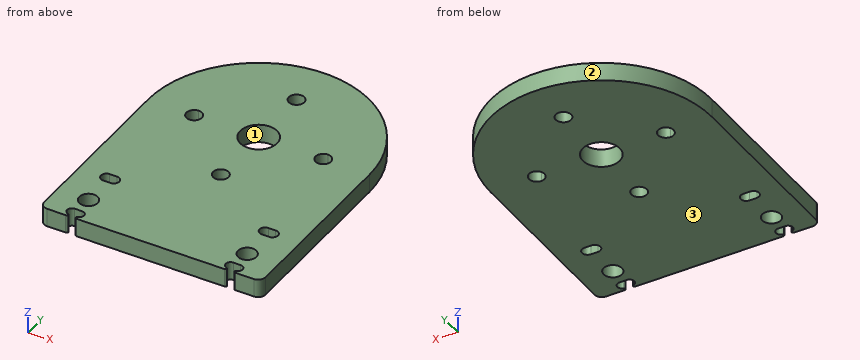
```python
from build123d import *

# Parameters (mm, degrees)
SKETCH1_R           = 2.5
BOSS_EXTRUDE1_DEPTH = 2.5
SKETCH2_R           = 5
CUT_EXTRUDE1_DEPTH  = 5
FILLET1_R           = 0.5
FILLET2_R           = 2


with BuildPart() as part:
    # Sketch1 → Boss-Extrude1 (new, symmetric)
    # profile 1 of 2: a face of its own
    with BuildSketch(Plane.XY):
        with BuildLine():
            Line((-30, 25), (-30, -25))
            Line((-30, -25), (-22.5, -25))
            Line((-22.5, -25), (-22.5, -24.3))
            ThreePointArc((-22.5, -24.3), (-23.8, -23), (-22.5, -21.7))
            Line((-22.5, -21.7), (-20.5, -21.7))
            ThreePointArc((-20.5, -21.7), (-19.2, -23), (-20.5, -24.3))
            Line((-20.5, -24.3), (-20.5, -25))
            Line((-20.5, -25), (20.5, -25))
            Line((20.5, -25), (20.5, -24.3))
            ThreePointArc((20.5, -24.3), (19.2, -23), (20.5, -21.7))
            Line((20.5, -21.7), (22.5, -21.7))
            ThreePointArc((22.5, -21.7), (23.8, -23), (22.5, -24.3))
            Line((22.5, -24.3), (22.5, -25))
            Line((22.5, -25), (30, -25))
            Line((30, -25), (30, 25))
            Line((30, 25), (-30, 25))
        make_face()
        with Locations((-21.5, -17)):
            Circle(SKETCH1_R, mode=Mode.SUBTRACT)
        with BuildLine():
            Line((-22.5, -5.5), (-20.5, -5.5))
            ThreePointArc((-20.5, -5.5), (-19, -7), (-20.5, -8.5))
            Line((-20.5, -8.5), (-22.5, -8.5))
            ThreePointArc((-22.5, -8.5), (-24, -7), (-22.5, -5.5))
        make_face(mode=Mode.SUBTRACT)
        with Locations((21.5, -17)):
            Circle(SKETCH1_R, mode=Mode.SUBTRACT)
        with BuildLine():
            ThreePointArc((20.5, -8.5), (19, -7), (20.5, -5.5))
            Line((20.5, -5.5), (22.5, -5.5))
            ThreePointArc((22.5, -5.5), (24, -7), (22.5, -8.5))
            Line((22.5, -8.5), (20.5, -8.5))
        make_face(mode=Mode.SUBTRACT)
    # profile 2 of 2: a face of its own
    with BuildSketch(Plane.XY):
        with BuildLine():
            ThreePointArc((30, 25), (0, 55), (-30, 25))
            Line((-30, 25), (30, 25))
        make_face()
    extrude(amount=BOSS_EXTRUDE1_DEPTH, both=True)

    # Sketch2 → Cut-Extrude1 (cut)
    with BuildSketch(Plane.XY.offset(2.5)):
        with Locations((0, 25)):
            Circle(SKETCH2_R)
        with BuildLine():
            ThreePointArc((-17.5, 27.1), (-19.6, 25), (-17.5, 22.9))
            Line((-17.5, 22.9), (-17.5, 27.1))
        make_face()
        with BuildLine():
            Line((-17.5, 27.1), (-17.5, 22.9))
            ThreePointArc((-17.5, 22.9), (-16.01507576, 23.51507576), (-15.4, 25))
            ThreePointArc((-15.4, 25), (-16.01507576, 26.48492424), (-17.5, 27.1))
        make_face()
        with BuildLine():
            ThreePointArc((17.5, 27.1), (15.4, 25), (17.5, 22.9))
            Line((17.5, 22.9), (17.5, 27.1))
        make_face()
        with BuildLine():
            Line((17.5, 27.1), (17.5, 22.9))
            ThreePointArc((17.5, 22.9), (18.98492424, 23.51507576), (19.6, 25))
            ThreePointArc((19.6, 25), (18.98492424, 26.48492424), (17.5, 27.1))
        make_face()
        with BuildLine():
            ThreePointArc((-2.1, 42.5), (0, 40.4), (2.1, 42.5))
            Line((2.1, 42.5), (-2.1, 42.5))
        make_face()
        with BuildLine():
            Line((-2.1, 42.5), (2.1, 42.5))
            ThreePointArc((2.1, 42.5), (0, 44.6), (-2.1, 42.5))
        make_face()
        with BuildLine():
            ThreePointArc((-2.1, 7.5), (0, 5.4), (2.1, 7.5))
            Line((2.1, 7.5), (-2.1, 7.5))
        make_face()
        with BuildLine():
            Line((-2.1, 7.5), (2.1, 7.5))
            ThreePointArc((2.1, 7.5), (0, 9.6), (-2.1, 7.5))
        make_face()
    extrude(amount=-CUT_EXTRUDE1_DEPTH, mode=Mode.SUBTRACT)

    # Fillet1
    # the kernel refuses this fillet: 0.5 mm, written as the material it takes off along each edge
    with BuildSketch(Plane(origin=(22.5, -25, -3.75), x_dir=(1, 0, 0), z_dir=(0, 0, 1))) as fillet1_piece_1:
        with BuildLine():
            CenterArc((FILLET1_R, FILLET1_R), FILLET1_R, 180, 90)
            Line((0, FILLET1_R), (0, 0))
            Line((0, 0), (FILLET1_R, 0))
        make_face()
    extrude(amount=7.5, mode=Mode.SUBTRACT)
    with BuildSketch(Plane(origin=(20.5, -25, -3.75), x_dir=(-1, 0, 0), z_dir=(0, 0, 1)), Plane(origin=(-20.5, -25, -3.75), x_dir=(0, 1, 0), z_dir=(0, 0, 1)), Plane(origin=(-22.5, -25, -3.75), x_dir=(-1, 0, 0), z_dir=(0, 0, 1))) as fillet1_piece_2:
        with BuildLine():
            CenterArc((FILLET1_R, -FILLET1_R), FILLET1_R, 90, 90)
            Line((0, -FILLET1_R), (0, 0))
            Line((0, 0), (FILLET1_R, 0))
        make_face()
    extrude(amount=7.5, mode=Mode.SUBTRACT)
    with BuildSketch(Plane(origin=(22.5, -24.3, -3.572904116), x_dir=(0, -1, 0), z_dir=(0, 0, 1))) as fillet1_piece_3:
        with BuildLine():
            CenterArc((0.429161647, 0.5), FILLET1_R, 196.127620213, 73.872379787)
            ThreePointArc((-0.051161033, 0.361111111), (-0.012853805, 0.182358634), (0, 0))
            Line((0, 0), (0.429161647, 0))
        make_face()
    extrude(amount=7.145808233, mode=Mode.SUBTRACT)
    with BuildSketch(Plane(origin=(20.5, -24.3, -3.572904116), x_dir=(-0.9901124580598394, 0.1402758724610287, 0), z_dir=(0, 0, 1))) as fillet1_piece_4:
        with BuildLine():
            CenterArc((0.434855205, 0.495056229), FILLET1_R, 188.063810107, 73.872379787)
            Line((-0.060201024, 0.424918293), (0, 0))
            ThreePointArc((0, 0), (0.182358634, 0.012853805), (0.364717268, 0))
        make_face()
    extrude(amount=7.145808233, mode=Mode.SUBTRACT)
    with BuildSketch(Plane(origin=(-20.5, -24.3, -3.572904116), x_dir=(0.9901124580598384, 0.14027587246103554, 0), z_dir=(0, 0, 1))) as fillet1_piece_5:
        with BuildLine():
            CenterArc((0.434855205, -0.495056229), FILLET1_R, 98.063810107, 73.872379787)
            Line((-0.060201024, -0.424918293), (0, 0))
            ThreePointArc((0, 0), (0.182358634, -0.012853805), (0.364717268, 0))
        make_face()
    extrude(amount=7.145808233, mode=Mode.SUBTRACT)
    with BuildSketch(Plane(origin=(-22.5, -24.3, -3.572904116), x_dir=(0, -1, 0), z_dir=(0, 0, 1))) as fillet1_piece_6:
        with BuildLine():
            CenterArc((0.429161647, -0.5), FILLET1_R, 90, 73.872379787)
            ThreePointArc((-0.051161033, -0.361111111), (-0.012853805, -0.182358634), (0, 0))
            Line((0, 0), (0.429161647, 0))
        make_face()
    extrude(amount=7.145808233, mode=Mode.SUBTRACT)

    # Fillet2
    fillet2_edges = [part.edges().sort_by_distance(p)[0] for p in [
        (-30, -25, 0),
        (30, -25, 0),
    ]]
    fillet(fillet2_edges, radius=FILLET2_R)


solid = part.part
```
Can you work these out from the model? Positions are in its coordinate system, mm. Face numbers are marked on the shaded views. Round coordinates to 2 decimals unless told otherwise and drop trailing zeros. Loops run counter-clockwise (first coordinate to the right, second up) from the corner with the lowest first, then second, coordinate; pieces in that order, holes last. Notation, with made-up numbers: (-35, 45.5) -> (-17, 45.5) arc R16 ccw to (-17, 70.5) -> close; hole circle Ø2 at (81, 74.25). An arc over 180 degrees is marked (long way). Answer in a Markdown table with one row per item.
Item 1: Suppose I cut it at D-D, the plane x = 16.5. List the corners of the cut face in (y, z) for me, plus the area to 3 significant figures.
Answer block:
| item | result |
|---|---|
| outline | (-25, -2.5) -> (23.15, -2.5) -> (23.15, 2.5) -> (-25, 2.5) -> close; (26.85, -2.5) -> (50.05, -2.5) -> (50.05, 2.5) -> (26.85, 2.5) -> close |
| area | 357 mm² |
Item 2: We'd pull the mould along X, two halves only. Please class the marked faces 1, 2 and 3: released by +X, released by -X, zero draft, split by the parting line, or undercut.
Answer block:
| item | result |
|---|---|
| face 1 | undercut |
| face 2 | split by the parting line |
| face 3 | zero draft |
Item 3: Suppose I cut it at A-A, the plane y = 7.5. List the corners of the cut face in (x, z) for me, plus the area to 3 significant figures.
Answer block:
| item | result |
|---|---|
| outline | (-30, -2.5) -> (-2.1, -2.5) -> (-2.1, 2.5) -> (-30, 2.5) -> close; (2.1, -2.5) -> (30, -2.5) -> (30, 2.5) -> (2.1, 2.5) -> close |
| area | 279 mm² |
Item 4: If I drill on probe 1 along Y at (x, z) = (0, 1.3); probe 2 along Y at (x, z) = (-21, 0.05); probe 3 along Y at (x, z) = (-22, 0.5), over which ranges is the centre line in solid material (lowest first)?
Answer block:
| item | result |
|---|---|
| probe 1 | -25 to 5.4, 9.6 to 20, 30 to 40.4, 44.6 to 55 |
| probe 2 | -21.7 to -19.45, -14.55 to -8.5, -5.5 to 46.42 |
| probe 3 | -21.7 to -19.45, -14.55 to -8.5, -5.5 to 45.4 |
Item 5: Will these pins go through, and if not, where does the flat tip stop? P1, Ø3, axis at x = 18.5, z = 0, coming from the +Y side; P2, Ø1, axis at x = 21, z = 0, coming from the +Y side; P3, Ø5.5, axis at x = 0, y = 42.5, coming from the -Z side; P4, Ø1.6, axis at x = -21, z = 0.5, coming from the -Y side.
Answer block:
| item | result |
|---|---|
| P1 | y = 49.72 |
| P2 | y = 46.9 |
| P3 | z = -2.5 |
| P4 | y = -24.96 |
Item 6: Suppose I cut it at B-B, the plane x = 0. List the corners of the cut face in (y, z) for me.
Answer block:
| item | result |
|---|---|
| outline | (-25, -2.5) -> (5.4, -2.5) -> (5.4, 2.5) -> (-25, 2.5) -> close; (9.6, -2.5) -> (20, -2.5) -> (20, 2.5) -> (9.6, 2.5) -> close; (30, -2.5) -> (40.4, -2.5) -> (40.4, 2.5) -> (30, 2.5) -> close; (44.6, -2.5) -> (55, -2.5) -> (55, 2.5) -> (44.6, 2.5) -> close |
Item 7: Suppose I cut it at C-C, the plane y = -16. List the corners of the cut face in (x, z) for me, plus the area to 3 significant figures.
Answer block:
| item | result |
|---|---|
| outline | (-30, -2.5) -> (-23.79, -2.5) -> (-23.79, 2.5) -> (-30, 2.5) -> close; (-19.21, -2.5) -> (19.21, -2.5) -> (19.21, 2.5) -> (-19.21, 2.5) -> close; (23.79, -2.5) -> (30, -2.5) -> (30, 2.5) -> (23.79, 2.5) -> close |
| area | 254 mm² |
